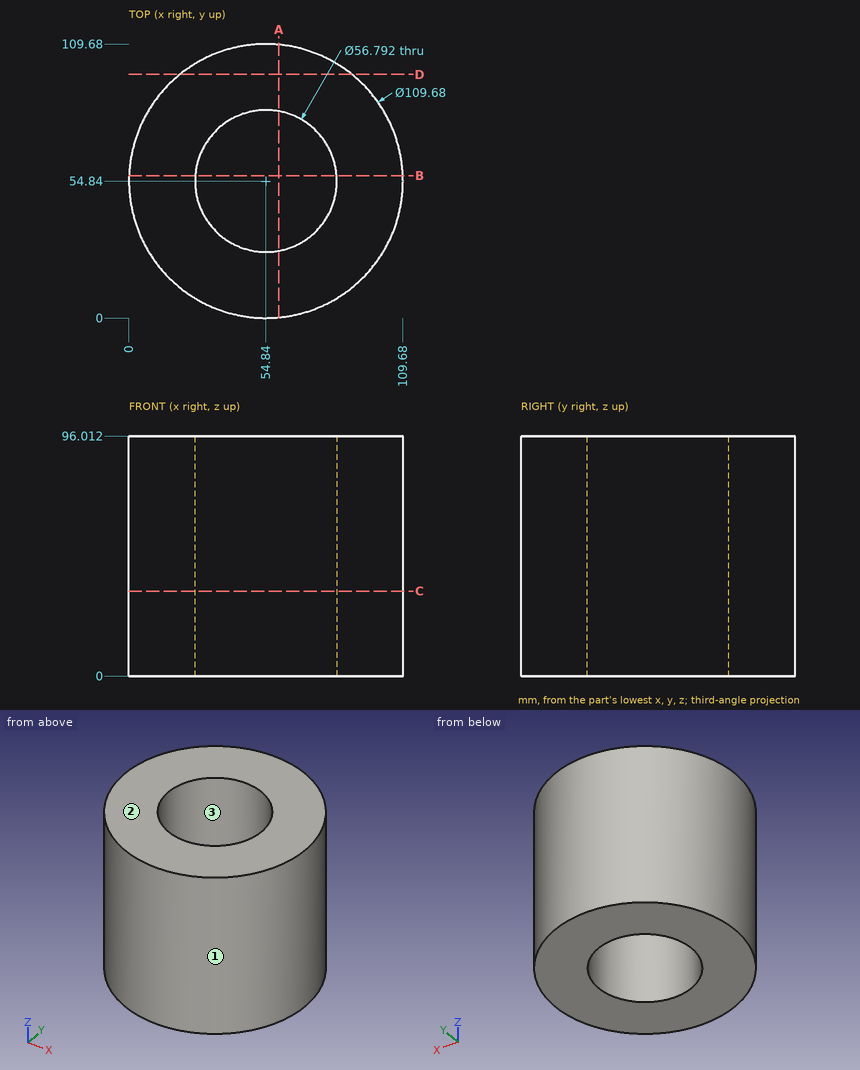
Answer from the drawing. Dimensions are ordinates in mm from the lowest x, y and z of the part. Coordinates: 2 decimals unless noted, no trailing zeros. Write each loop counter-clockwise with the first axis right and the second up, starting at its lowest first coordinate (ties: lowest second). Pieces come first, ordered by that corner, then holes. Notation, with made-up numbers: (62, 62) - (103, 62) arc R19 cw to (103, 86) - close; hole circle Ø11 at (66.5, 56). An arc over 180 degrees is marked (long way). Return JSON: item names as keys, results as strings. Group by question number.
Q1. For a pull along Y with two mould halves and no side action, classify the marked faces 1, 2 and 3 as +Y half, -Y half, draft (parallel to the pull), parting line (faces both ways), or undercut.
Q2. Flat-ended cylindrical pins translate along their axes: pin 1 Ø1.5 at (y, z) = (18.5, 67.5) entering from +X; pin 2 Ø5 at (x, z) = (80, 55.5) entering from -Y; pin 3 Ø1 at (x, z) = (62.5, 36) entering from -Y. Find the tip coordinate at first contact, or state that the pin passes through.
Q3. The part is cut by section D-D on y = 97.5. Write down the section's boundary in (x, z), and give its area (3 significant figures).
Q4. The part is cut by section C-C on z = 34. Write down the section's boundary in (x, y).
Q5. The part is cut by section A-A on x = 60. Write down the section's boundary in (y, z).
Q6. The part is cut by section B-B on y = 57. Write down the section's boundary in (x, z).
Q7. Find the intervals of material crossed by line 1 along Y through (x, z) = (56, 57.5); line 2 along X through (y, z) = (51.5, 83.5); line 3 along Y through (x, z) = (42.5, 6) (1 decimal), in increasing order. Write a range as [from, to].
Evaluation:
{
 "1": {"face 1": "parting line", "face 2": "draft", "face 3": "undercut"},
 "2": {"pin 1": "stops at x = 96.56", "pin 2": "stops at y = 4.9", "pin 3": "stops at y = 0.47"},
 "3": {"outline": "(20.38, 0) - (89.3, 0) - (89.3, 96.01) - (20.38, 96.01) - close", "area": "6,620 mm2"},
 "4": {"outline": "circle Ø109.68 at (54.84, 54.84); hole circle Ø56.79 at (54.84, 54.84)"},
 "5": {"outline": "(0.24, 0) - (26.92, 0) - (26.92, 96.01) - (0.24, 96.01) - close; (82.76, 0) - (109.44, 0) - (109.44, 96.01) - (82.76, 96.01) - close"},
 "6": {"outline": "(0.04, 0) - (26.53, 0) - (26.53, 96.01) - (0.04, 96.01) - close; (83.15, 0) - (109.64, 0) - (109.64, 96.01) - (83.15, 96.01) - close"},
 "7": {"line 1": "y = [0.01, 26.47], [83.21, 109.67]", "line 2": "x = [0.1, 26.64], [83.04, 109.58]", "line 3": "y = [1.4, 29.3], [80.4, 108.3]"}
}
